Build history of the part. All positions in model axes, mm. Give positions to 0.01 mm unless a question says otherwise; leave off trailing zeros. Loops run counter-clockwise (first coordinate to the right, second up) from the corner with the lowest first, then second, coordinate; pieces in that order, holes last. Notation, with made-up numbers: (74, 60.25) -> (87, 60.25) arc R32 cw to (87, 95.25) -> close; hole circle Ø2 at (40, -37.5). An arc over 180 degrees is marked (long way). Answer as a JSON object with one key per item and string values. Group by question number.
Q1. Wall check: probe 1 along Z at (x, y) = (3, 787.5); probe 2 along Z at (x, y) = (0.5, 894.5); probe 3 along X at (y, z) = (927.5, 24.5). Give the ranges that are in metal, low to high. Write a range as from..to.
Q2. Drop flat-ended pins along their axis: pin 1 (4 mm diameter, centred on y = 745.5, z = -9.5, fed in from -X); pin 2 (1 mm diameter, centred on x = 14, z = 7.5, fed in from +Y); pin 3 (6 mm diameter, centred on y = 372, z = -16, fed in from +X). Give the stop position or say it passes through.
Q3. Band-saw the part on A-A, the plane y = 999. Write the cut outline in (x, z) (3 decimals), plus the area to 3 significant figures.
from build123d import *


with BuildPart() as part:
    # Sketch2 → Revolve1 (revolve)
    with BuildSketch(Plane.XY, mode=Mode.PRIVATE) as revolve1_sk:
        with BuildLine():
            Line((0, 1266.19), (0, 6.753760064))
            ThreePointArc((0, 6.753760064), (1.004358981, 7.115605787), (1.547169826, 8.034858568))
            ThreePointArc((1.547169826, 8.034858568), (20.581846727, 138.066176315), (28.575, 269.24))
            Line((28.575, 269.24), (28.575, 1266.19))
            Line((28.575, 1266.19), (0, 1266.19))
        make_face()
    revolve(revolve1_sk.sketch.rotate(Axis((0, 0, 0), (0, 1, 0)), 90), axis=Axis((0, 0, 0), (0, 1, 0)))

    # Sketch3 → Revolve2 (revolve)
    with BuildSketch(Plane.XY, mode=Mode.PRIVATE) as revolve2_sk:
        with BuildLine():
            Line((-28.575, 1312.926), (-28.575, 1266.19))
            Line((-28.575, 1266.19), (0, 1266.19))
            Line((0, 1266.19), (0, 1358.9))
            Line((0, 1358.9), (-16.6116, 1358.9))
            Line((-16.6116, 1358.9), (-18.669, 1359.451278669))
            Line((-18.669, 1359.451278669), (-18.872794116, 1358.690708673))
            Line((-18.872794116, 1358.690708673), (-17.219933754, 1358.247826074))
            ThreePointArc((-17.219933754, 1358.247826074), (-16.757242508, 1357.892790594), (-16.681118386, 1357.314570482))
            Line((-16.681118386, 1357.314570482), (-28.575, 1312.926))
        make_face()
    revolve(revolve2_sk.sketch.rotate(Axis((0, 1358.9, 0), (0, -1, 0)), 270), axis=Axis((0, 1358.9, 0), (0, -1, 0)))


solid = part.part
Worked answers:
{
 "1": {"probe 1": "-28.42..28.42", "probe 2": "-28.57..28.57", "probe 3": "-14.71..14.71"},
 "2": {"pin 1": "x = -27.57", "pin 2": "y = 1358.9", "pin 3": "x = 25.45"},
 "3": {"outline": "circle Ø57.15 at (0, 0)", "area": "2,570 mm2"}
}
